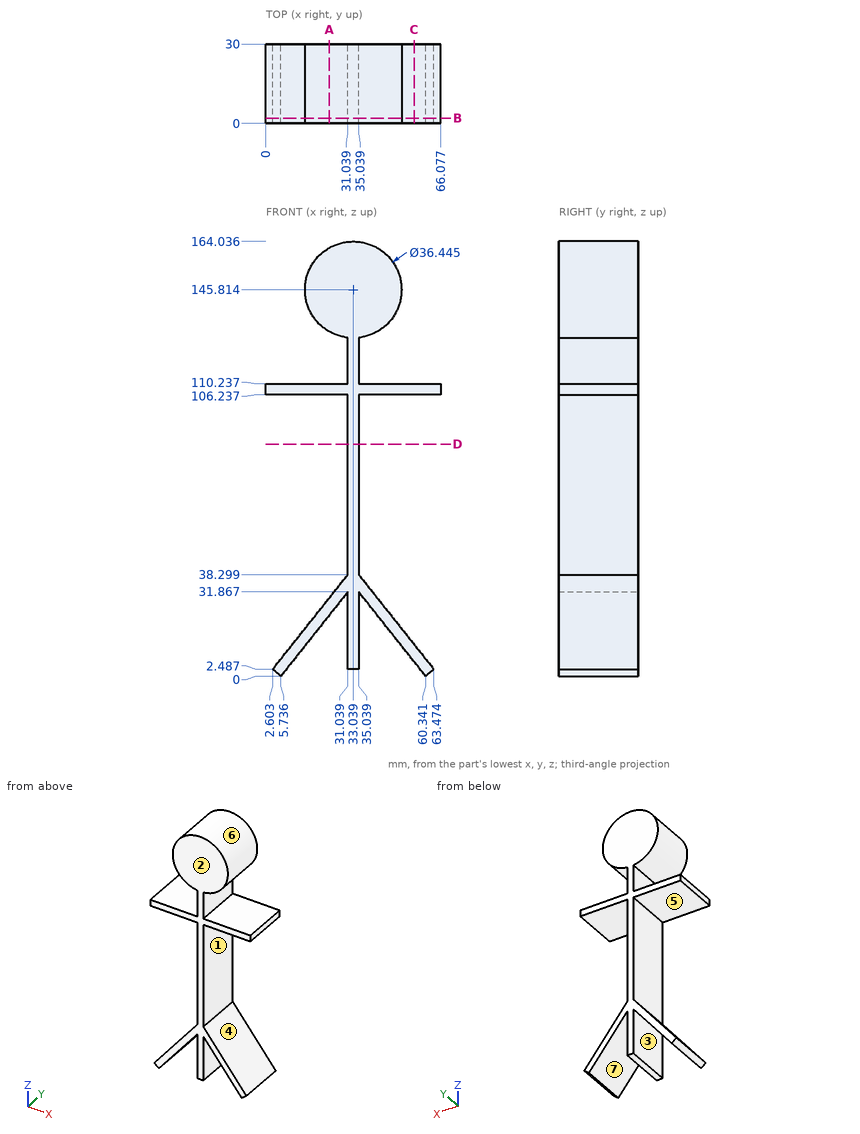
Verification items for this drawing (mm, ordinates from the low corner). A direction names the side the tool comes from. Round coordinates to 2 decimals unless told otherwise and drop trailing zeros. Order: outer loops, then holes, each group sorted by start corner. A loop starts at its lowest first (then second) coordinate and runs counter-clockwise, first axis right, second up. Notation, with made-up numbers: (6, -37.5) - (29, -37.5) arc R21 ccw to (29, -26.5) - close; hole circle Ø5 at (-1, 61.25). An arc over 180 degrees is marked (long way). Answer as CSV lines item,"result". Start each with the question number.
1) Depth check by flat-ended pin: pin 1 (1.2 mm diameter, centred on x = 33, y = 8.5, fed in from -Z); pin 2 (12 mm diameter, centred on y = 8.5, z = 115.5, fed in from -X); pin 3 (14.5 mm diameter, centred on y = 20, z = 23.5, fed in from -X); pin 4 (14 mm diameter, centred on y = 15.5, z = 123, fed in from -X) (1 decimal). Enter the tip coordinate at first touch or a pass-through.
2) Section check A-A (x = 24). Record the cut outline in (y, z) (1 decimal).
3) Section check C-C (x = 56). Record the cut outline in (y, z), then the cut area to 3 significant figures.
4) Draft check along X on the marked faces 1, 2 and 3. Enter one of: +X half, -X half, draft (parallel to the pull), parting line (faces both ways), or undercut.
5) Tool access check on the marked faces 4, 5, 6 and 7. Record the directions out of +Z, -Z, +X, -X, +Y, -Y that give a thin tool (end or side, any length) a straight path to the whole face; none if there is none.
6) Section check D-D (z = 87.5). Record the cut outline in (x, y), then the cut area to 3 significant figures.
7) Section check B-B (y = 2). Record the cut outline in (x, z) (1 decimal).
8) Scan lines: probe 1 along Z at (x, y) = (19, 4.25) (1 decimal); probe 2 along Z at (x, y) = (47, 8.75) (1 decimal); probe 3 along X at (y, z) = (16, 24.5) (1 decimal). Record each from-to range of solid material in increasing order.
Determined:
1,pin 1,"z = 2.49"
1,pin 2,"x = 0"
1,pin 3,"x = 13.53"
1,pin 4,"x = 24"
2,outline,"(0, 23) - (30, 23) - (30, 29.4) - (0, 29.4) - close; (0, 106.2) - (30, 106.2) - (30, 110.2) - (0, 110.2) - close; (0, 130) - (30, 130) - (30, 161.6) - (0, 161.6) - close"
3,outline,"(0, 5.47) - (30, 5.47) - (30, 11.9) - (0, 11.9) - close; (0, 106.24) - (30, 106.24) - (30, 110.24) - (0, 110.24) - close"
3,area,"313 mm^2"
4,face 1,"+X half"
4,face 2,"draft"
4,face 3,"undercut"
5,face 4,"+X, +Y, -Y"
5,face 5,"-X, +Y, -Y"
5,face 6,"+Y, -Y"
5,face 7,"-Z, +Y, -Y"
6,outline,"(31.04, 0) - (35.04, 0) - (35.04, 30) - (31.04, 30) - close"
6,area,"120 mm^2"
7,outline,"(0, 106.2) - (31, 106.2) - (31, 38.3) - (2.6, 2.5) - (5.7, 0) - (31, 31.9) - (31, 2.5) - (35, 2.5) - (35, 31.9) - (60.3, 0) - (63.5, 2.5) - (35, 38.3) - (35, 106.2) - (66.1, 106.2) - (66.1, 110.2) - (35, 110.2) - (35, 127.7) arc R18.2 ccw (long way) to (31, 127.7) - (31, 110.2) - (0, 110.2) - close"
8,probe 1,"16.7 to 23.1, 106.2 to 110.2, 134.2 to 157.4"
8,probe 2,"16.8 to 23.2, 106.2 to 110.2, 134.1 to 157.5"
8,probe 3,"20.1 to 25.2, 31 to 35, 40.9 to 46"
